The listing builds one solid part. Answer for the finished solid, in the listing's coordinates (mm). Give positions to 0.01 mm unless a question says otherwise; leave off trailing zeros. Loops run counter-clockwise (first coordinate to the right, second up) from the corner with the lowest first, then second, coordinate; pieces in that order, holes last. Notation, with made-up numbers: (69.5, 9) - (125.5, 9) arc R18 ccw to (125.5, 24) - close; hole circle Ø2 at (-22, 9.5). An arc over 180 degrees is marked (long way). Answer in a Markdown table with one row per item. Add a question column.
Autodesk Inventor part; units mm, degrees
ref_plane "YZ Plane" through (0, 0, 0) normal (1, 0, 0) x (0, 1, 0)
ref_plane "XZ Plane" through (0, 0, 0) normal (0, 1, 0) x (-1, 0, 0)
ref_plane "XY Plane" through (0, 0, 0) normal (0, 0, 1) x (1, 0, 0)
sketch "Эскиз1" plane through (0, 0, 0) normal (0, 0, 1) x (1, 0, 0)
  line L0 (-145, 120) -> (145, 120)
  line L1 (145, 120) -> (145, -120)
  line L2 (145, -120) -> (-145, -120)
  line L3 (-145, -120) -> (-145, 120)
  line L4 (-145, 120) -> (145, -120) construction
  line L5 (145, 120) -> (-145, -120) construction
  point P0 (0, 0)
  dimension "d0" = 240
  dimension "d1" = 290
extrude "Пластина1" add sketch "Эскиз1" along normal blind 3
sketch "Эскиз2" plane through (0, 0, 3) normal (0, 0, 1) x (1, 0, 0)
  line L0 (12.5, 105) -> (-12.5, 105)
  line L1 (-12.5, 105) -> (-12.5, 115)
  line L2 (-12.5, 115) -> (12.5, 115)
  line L3 (12.5, 115) -> (12.5, 105)
  line L4 (122, -15.0105) -> (122, 14.9895)
  line L5 (122, 14.9895) -> (132, 14.9895)
  line L6 (132, 14.9895) -> (132, -15.0105)
  line L7 (132, -15.0105) -> (122, -15.0105)
  line L8 (122.0074, 94.9791) -> (132.0074, 94.9783)
  line L9 (132.0074, 94.9783) -> (132.0051, 64.9783)
  line L10 (132.0051, 64.9783) -> (122.0051, 64.9791)
  line L11 (122.0051, 64.9791) -> (122.0074, 94.9791)
  line L12 (12.5, -105) -> (12.5, -115)
  line L13 (12.5, -115) -> (-12.5, -115)
  line L14 (-12.5, -115) -> (-12.5, -105)
  line L15 (-12.5, -105) -> (12.5, -105)
  circle A0 centre (-107, 95) radius 1.5
  circle A1 centre (107, -95) radius 1.5
  circle A2 centre (107, 95) radius 1.5
  line L16 (122, -65) -> (132, -65)
  line L17 (132, -65) -> (132, -95)
  line L18 (132, -95) -> (122, -95)
  line L19 (122, -95) -> (122, -65)
  circle A3 centre (-107, -95) radius 1.5
  line L20 (-147, 125) -> (-147, -125)
  line L21 (-147, -125) -> (147, -125)
  line L22 (147, -125) -> (147, 125)
  line L23 (147, 125) -> (-147, 125)
  point P0 (0, 0)
extrude "Выдавливание1" cut sketch "Эскиз2" against normal through all contours L0 L1 L2 L3 | L4 L5 L6 L7 | L8 L9 L10 L11 | L12 L13 L14 L15 | A0 | A1 | A2 | L16 L17 L18 L19 | A3
equation "\"d2\" = Толщина"
equation "\"Радиус_гибки\" = Толщина"
equation "\"Ширина_просечки\" = Толщина"
equation "\"Глубина_просечки\" = 0.5 * Толщина"
equation "\"Размер_просечки\" = 4 * Толщина"
equation "\"Мин_остаток\" = 2 * Толщина"
equation "\"Радиус_перехода\" = Радиус_гибки"
equation "\"Радиус_Якоби\" = Радиус_гибки"
equation "\"Размер_зазора\" = Толщина"
properties part number "панель_с_электроникой"
(1) A cutting plane is placed at B-B on z = 1.6. Give the number of separate pieces and of enclosed holes in the cut face, plus the area to 3 significant figures.
(2) A cutting plane is placed at A-A on y = -79.5. Determine the outline of the cut face in (x, z), plus the area to 3 significant figures.
(3) Find the intervals of material crossed by line 1 along Y through (x, z) = (-107, 2); line 2 along X through (y, z) = (-6.5, 2.2); line 3 along Y through (x, z) = (6.5, 1.45), in increasing order. Write a range as [from, to].
Evaluation:
| question | item | result |
|---|---|---|
| 1 | separate pieces | 1 |
| 1 | enclosed holes | 9 |
| 1 | area | 68,200 mm² |
| 2 | outline | (-145, 0) - (122, 0) - (122, 3) - (-145, 3) - close; (132, 0) - (145, 0) - (145, 3) - (132, 3) - close |
| 2 | area | 840 mm² |
| 3 | line 1 | y = [-120, -96.5], [-93.5, 93.5], [96.5, 120] |
| 3 | line 2 | x = [-145, 122], [132, 145] |
| 3 | line 3 | y = [-120, -115], [-105, 105], [115, 120] |
